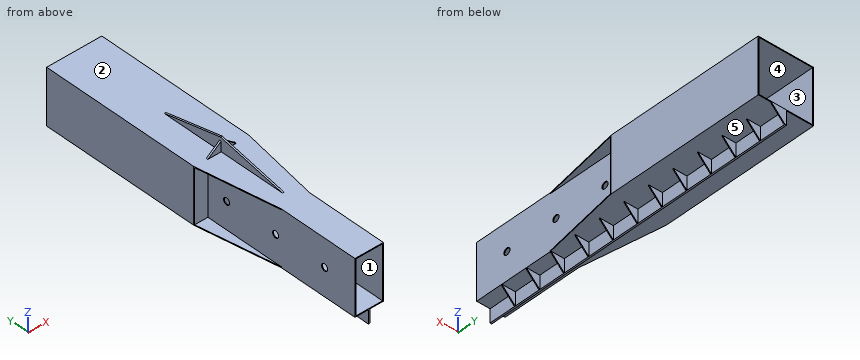
from build123d import *

# Parameters (mm, degrees)
F0_W           = 104.775
F0_H           = 104.775
F0_W_2         = 101.6
F0_H_2         = 101.6
F1_DEPTH       = 1.5875
F3_DEPTH       = 304.8
F5_DEPTH       = 304.8
F6_W           = 152.4
F6_H           = 1.5875
F7_DEPTH       = 25.4
F8_W           = 152.4
F8_H           = 1.5875
F9_DEPTH       = 25.4
F11_DEPTH      = 177.8
F12_W          = 3.175
F12_H          = 611.1875
F13_DEPTH      = 25.4
F14_R          = 6.35
F15_DEPTH      = 213.36
F16_W          = 25.4
F16_H          = 1.5875
F17_DEPTH      = 25.4
F19_DEPTH      = 1828.8
F20_W          = 1.5875
F20_H          = 245.0186535716
F21_DEPTH      = 25.4
F23_DEPTH      = 25.4
F24_W          = 1.5875
F24_H          = 19.05
F25_DEPTH      = 25.4
F25_DEPTH_BACK = 28.575
F27_DEPTH      = 25.4
F29_DEPTH      = 25.4


with BuildPart() as f1:
    # F0 (on Front) → F1 (new body)
    with BuildSketch(Plane.XZ):
        with Locations((-4.1154902428, 8.1752620383)):
            Rectangle(F0_W, F0_H)
        with Locations((-4.1154902428, 8.1752620383)):
            Rectangle(F0_W_2, F0_H_2, mode=Mode.SUBTRACT)
        with Locations((-4.1154902428, 8.1752620383)):
            Rectangle(F0_W_2, F0_H_2)
    extrude(amount=F1_DEPTH)

    # F2 (on face) → F3 (join)
    with BuildSketch(Plane(origin=(0, 0, 0), x_dir=(-1, 0, 0), z_dir=(0, 1, 0))):
        Polygon((-46.6845097572, 58.9752620383), (-48.2720097572, 60.5627620383), (-48.2720097572, -44.2122379617), (56.5029902428, -44.2122379617), (54.9154902428, -42.6247379617), (-46.6845097572, -42.6247379617), align=None)
        Polygon((56.5029902428, 60.5627620383), (-48.2720097572, 60.5627620383), (-46.6845097572, 58.9752620383), (54.9154902428, 58.9752620383), (54.9154902428, -42.6247379617), (56.5029902428, -44.2122379617), align=None)
    extrude(amount=F3_DEPTH)

    # F4 (on face) → F5 (join)
    with BuildSketch(Plane.XZ.offset(1.5875)):
        Polygon((-31.1029902428, 60.5627620383), (-31.1029902428, 35.1627620383), (-29.5154902428, 33.5752620383), (-29.5154902428, 58.9752620383), (21.2845097572, 58.9752620383), (21.2845097572, -17.2247379617), (22.8720097572, -18.8122379617), (22.8720097572, 60.5627620383), align=None)
        Polygon((-29.5154902428, 33.5752620383), (-31.1029902428, 35.1627620383), (-31.1029902428, -44.2122379617), (22.8720097572, -44.2122379617), (22.8720097572, -18.8122379617), (21.2845097572, -17.2247379617), (21.2845097572, -42.6247379617), (-29.5154902428, -42.6247379617), align=None)
    extrude(amount=F5_DEPTH)

    # F6 (on face) → F7 (join)
    with BuildSketch(Plane(origin=(-31.1029902428, 0, 0), x_dir=(0, -1, 0), z_dir=(-1, 0, 0))):
        with Locations((77.7875, 59.7690120383)):
            Rectangle(F6_W, F6_H)
        with Locations((77.7875, -43.4184879617)):
            Rectangle(F6_W, F6_H)
    extrude(amount=F7_DEPTH)

    # F8 (on face) → F9 (join)
    with BuildSketch(Plane.YZ.offset(22.8720097572)):
        with Locations((-77.7875, 59.7690120383)):
            Rectangle(F8_W, F8_H)
        with Locations((-77.7875, -43.4184879617)):
            Rectangle(F8_W, F8_H)
    extrude(amount=F9_DEPTH)

    # F10 (on face) → F11 (cut)
    with BuildSketch(Plane.XY.offset(60.5627620383)):
        Polygon((-31.1029902428, -153.9875), (-56.5029902428, 0), (-56.5029902428, -153.9875), align=None)
        Polygon((48.2720097572, -153.9875), (48.2720097572, 0), (22.8720097572, -153.9875), align=None)
    extrude(amount=-F11_DEPTH, mode=Mode.SUBTRACT)

    # F12 (on face) → F13 (join)
    with BuildSketch(Plane(origin=(0, 0, -44.2122379617), x_dir=(1, 0, 0), z_dir=(0, 0, -1))):
        with Locations((-4.1154902428, 0.79375)):
            Rectangle(F12_W, F12_H)
    extrude(amount=F13_DEPTH)

    # F14 (on face) → F15 (cut)
    with BuildSketch(Plane(origin=(-31.1029902428, 0, 0), x_dir=(0, -1, 0), z_dir=(-1, 0, 0))):
        with Locations((40.4604896903, 8.1752620383)):
            Circle(F14_R)
        with Locations((142.0604896903, 8.1752620383)):
            Circle(F14_R)
        with Locations((243.6604896903, 8.1752620383)):
            Circle(F14_R)
    extrude(amount=-F15_DEPTH, mode=Mode.SUBTRACT)

    # F16 (on face) → F17 (join)
    with BuildSketch(Plane(origin=(0, 0, -44.2122379617), x_dir=(1, 0, 0), z_dir=(0, 0, -1))):
        with Locations((10.1720097572, -304.00625)):
            Rectangle(F16_W, F16_H)
        with Locations((10.1720097572, -253.20625)):
            Rectangle(F16_W, F16_H)
        with Locations((10.1720097572, -202.40625)):
            Rectangle(F16_W, F16_H)
        with Locations((10.1720097572, -151.60625)):
            Rectangle(F16_W, F16_H)
        with Locations((10.1720097572, -100.80625)):
            Rectangle(F16_W, F16_H)
        with Locations((10.1720097572, -50.00625)):
            Rectangle(F16_W, F16_H)
        with Locations((10.1720097572, 0.79375)):
            Rectangle(F16_W, F16_H)
        with Locations((10.1720097572, 102.39375)):
            Rectangle(F16_W, F16_H)
        with Locations((10.1720097572, 51.59375)):
            Rectangle(F16_W, F16_H)
        with Locations((10.1720097572, 153.19375)):
            Rectangle(F16_W, F16_H)
        with Locations((10.1720097572, 203.99375)):
            Rectangle(F16_W, F16_H)
        with Locations((10.1720097572, 254.79375)):
            Rectangle(F16_W, F16_H)
    extrude(amount=F17_DEPTH)

    # F18 (on face) → F19 (cut)
    with BuildSketch(Plane(origin=(0, 304.8, 0), x_dir=(-1, 0, 0), z_dir=(0, 1, 0))):
        Polygon((-22.8720097572, -69.6122379617), (2.3494476918, -69.6122379617), (-22.8720097572, -44.2122379617), align=None)
    extrude(amount=-F19_DEPTH, mode=Mode.SUBTRACT)

    # F20 (on face) → F21 (join)
    with BuildSketch(Plane.XY.offset(60.5627620383)):
        with Locations((-4.9092402428, -5.9108771384)):
            Rectangle(F20_W, F20_H)
        with Locations((-3.3217402428, -5.9108771384)):
            Rectangle(F20_W, F20_H)
    extrude(amount=F21_DEPTH)

    # F22 (on face) → F23 (cut)
    with BuildSketch(Plane(origin=(-5.7029902428, 0, 0), x_dir=(0, -1, 0), z_dir=(-1, 0, 0))):
        Polygon((-116.5984496474, 85.9627620383), (-116.5984496474, 60.5627620383), (0, 85.9627620383), align=None)
        Polygon((128.4202039242, 85.9627620383), (0, 85.9627620383), (128.4202039242, 60.5627620383), align=None)
    extrude(amount=-F23_DEPTH, mode=Mode.SUBTRACT)

    # F24 (on face) → F25 (join, two sides)
    with BuildSketch(Plane(origin=(-5.7029902428, 0, 0), x_dir=(0, -1, 0), z_dir=(-1, 0, 0))) as f25_sk:
        with Locations((-0.79375, 70.0877620383)):
            Rectangle(F24_W, F24_H)
        with Locations((0.79375, 70.0877620383)):
            Rectangle(F24_W, F24_H)
    extrude(amount=F25_DEPTH)
    extrude(f25_sk.sketch, amount=-F25_DEPTH_BACK)

    # F26 (on face) → F27 (cut)
    with BuildSketch(Plane.XZ.offset(1.5875)):
        Polygon((-31.1029902428, 60.5627620383), (-5.7029902428, 79.6127620383), (-31.1029902428, 79.6127620383), align=None)
    extrude(amount=-F27_DEPTH, mode=Mode.SUBTRACT)

    # F28 (on face) → F29 (cut)
    with BuildSketch(Plane.XZ.offset(1.5875)):
        Polygon((22.8720097572, 79.6127620383), (-2.5279902428, 79.6127620383), (22.8720097572, 60.5627620383), align=None)
    extrude(amount=-F29_DEPTH, mode=Mode.SUBTRACT)


solid = f1.part
Design review of the part built by this model. Coordinates are the model's own, in mm. Face numbers are marked on the shaded views. A direction names the side the tool comes from. Round coordinates to 2 decimals unless told otherwise and drop trailing zeros. Order: outer loops, then holes, each group sorted by start corner. A loop starts at its lowest first (then second) coordinate and runs counter-clockwise, first axis right, second up. Notation, with made-up numbers: M -21.5,68.25 L 31.5,68.25 A22 cw 31.5,86.25 Z; hole C 50,0 d5. An arc over 180 degrees is marked long. Answer as CSV lines item,"result". Start each with the question number.
1) Add section A-A (y = -169). Give the boundary of the cut face in (x, z).
2) Wall thickness on line 1 along X through (y, z) = (-36, -41); line 2 along Z through (x, y) = (18, -22.5); line 3 along X through (y, z) = (153, -4): over which ranges is each line inside the solid? List them lowest first. Write a range as [from, to].
3) Tool access review of the marked faces 1, 2 and 3: name each direction out of +Z, -Z, +X, -X, +Y, -Y from which nothing blocks a thin tool from reaching the whole face with its end or side.
4) Add section B-B (z = -26.5). Give the boundary of the cut face in (x, y).
5) The part is to be moulded in two halves that separate along Y. For the marked faces 4 and 5, say which applies: +Y half, -Y half, draft (parallel to the pull), parting line (faces both ways), or undercut.
6) Add section C-C (y = 247). Give the boundary of the cut face in (x, z), then the cut area to 3 significant figures.
7) Add section D-D (z = 67). Give the boundary of the cut face in (x, y).
8) For pin 1 Ø20 at (x, y) = (-47, -72) entering from +Z; pin 2 Ø5 at (y, z) = (-81, 29.5) entering from -X; pin 3 Ø20.5 at (y, z) = (-166.5, -53.5) entering from +X, all flat-tipped, find the tip position at first contact; note any pin that passes through.
Resolved:
1,outline,"M -31.1,-44.21 L -5.7,-44.21 L -5.7,-69.61 L -2.53,-69.61 L -2.53,-44.21 L 22.87,-44.21 L 22.87,60.56 L -31.1,60.56 Z; hole M -29.52,-42.62 L 21.28,-42.62 L 21.28,58.98 L -29.52,58.98 Z"
2,line 1,"[-31.1, -29.52], [21.28, 22.87]"
2,line 2,"[-44.21, -42.62], [58.98, 60.56]"
2,line 3,"[-56.5, -54.92], [46.68, 48.27]"
3,face 1,"-Y"
3,face 2,"+Z"
3,face 3,"+Y"
4,outline,"M -56.5,0 L -56.24,-1.59 L -31.1,-1.59 L -31.1,-306.39 L -29.52,-306.39 L -29.52,-1.59 L 21.28,-1.59 L 21.28,-306.39 L 22.87,-306.39 L 22.87,-1.59 L 48.01,-1.59 L 48.27,0 L 48.27,304.8 L 46.68,304.8 L 46.68,0 L -54.92,0 L -54.92,304.8 L -56.5,304.8 Z"
5,face 4,"draft"
5,face 5,"undercut"
6,outline,"M -56.5,-44.21 L -5.7,-44.21 L -5.7,-69.61 L -2.53,-69.61 L -2.53,-44.21 L 48.27,-44.21 L 48.27,60.56 L -56.5,60.56 Z; hole M -54.92,-42.62 L 46.68,-42.62 L 46.68,58.98 L -54.92,58.98 Z"
6,area,"736 mm^2"
7,outline,"M -22.52,-1.59 L -5.7,-1.59 L -5.7,-95.87 L -2.53,-95.87 L -2.53,-1.59 L 14.29,-1.59 L 14.29,1.59 L -2.53,1.59 L -2.53,87.05 L -5.7,87.05 L -5.7,1.59 L -22.52,1.59 Z"
8,pin 1,"z = 60.56"
8,pin 2,"x = -31.1"
8,pin 3,"x = 22.87"
